Could you check a few things on this drawing? It's one solid part, dimensions in mm from its lowest x, y, z. Coordinates: 2 decimals unless noted, no trailing zeros. Order: outer loops, then holes, each group sorted by start corner. A loop starts at its lowest first (then second) coordinate and runs counter-clockwise, first axis right, second up. Notation, with made-up numbers: (52, 0.25) -> (94, 0.25) arc R20 cw to (94, 16.25) -> close; hole circle Ø4 at (65.25, 46.25). An arc over 180 degrees is marked (long way). Answer as CSV lines item,"result".
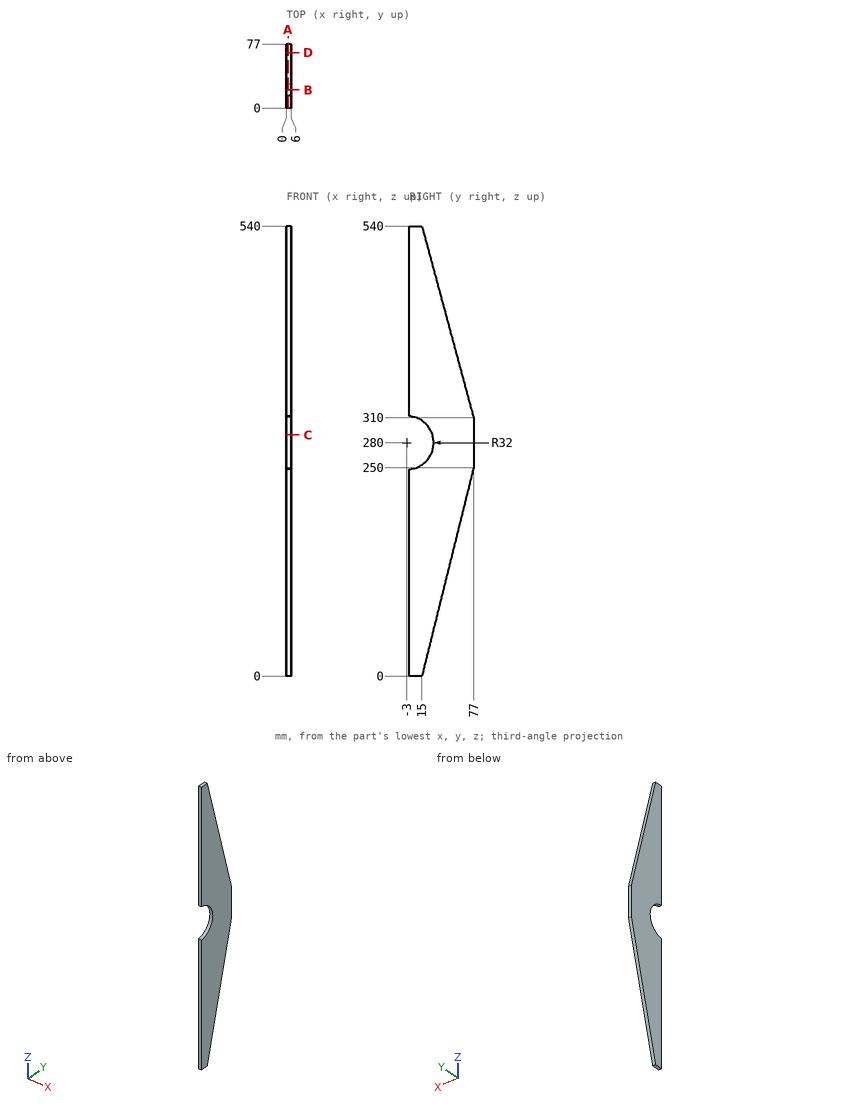
Q1. If I drill on line 1 (Z direction, x = 4.8, y = 8.5); line 2 (Z direction, x = 0.6, y = 11); line 3 (Y direction, x = 5.6, z = 274), over which ranges is the centre line in solid material (lowest first)?
Solution:
line 1,"0 to 250.14, 309.86 to 540"
line 2,"0 to 251.23, 308.77 to 540"
line 3,"28.43 to 77"
Q2. Imagine slicing it at D-D (y = 66.5). List the corners of the cut face in (x, z) for me, and give its area (3 significant figures).
Solution:
outline,"(0, 207.66) -> (6, 207.66) -> (6, 348.95) -> (0, 348.95) -> close"
area,"848 mm2"
Q3. Imagine slicing it at A-A (x = 1.95). List the corners of the cut face in (y, z) for me.
Solution:
outline,"(0, 0) -> (15, 0) -> (77, 250) -> (77, 310) -> (15, 540) -> (0, 540) -> (0, 311.86) arc R32 cw to (0, 248.14) -> close"
Q4. Imagine slicing it at B-B (y = 22). List the corners of the cut face in (x, z) for me.
Solution:
outline,"(0, 28.23) -> (6, 28.23) -> (6, 260.03) -> (0, 260.03) -> close; (0, 299.97) -> (6, 299.97) -> (6, 514.03) -> (0, 514.03) -> close"
Q5. Imagine slicing it at C-C (z = 289.5). List the corners of the cut face in (x, y) for me.
Solution:
outline,"(0, 27.56) -> (6, 27.56) -> (6, 77) -> (0, 77) -> close"
